Autodesk Fusion 360 part; units mm, degrees
sketch "Sketch1" plane through (0, 0, 0) normal (0, 1, 0) x (1, 0, 0)
  line L0 (0, 0) -> (39, 0)
  line L1 (0, 0) -> (-39, 0)
  line L2 (39, 0) -> (39, -36)
  line L3 (-39, -36) -> (39, -36)
  line L4 (-39, 0) -> (-49, -5.7735)
  line L5 (-39, 0) -> (1.8239, 0) construction
  line L6 (-49, -5.7735) -> (-49, -17.7735)
  line L7 (-49, -17.7735) -> (-39, -36)
  dimension "d1" = 39
  dimension "d2" = 39
  dimension "d4" = 36
  dimension "d5" = 36
  dimension "d8" = 12
extrude "Extrude1" add sketch "Sketch1" along normal mid plane 60
sketch "Sketch2" plane through (0, 0, 0) normal (0, 0, 1) x (1, 0, 0)
  line L0 (39, -30) -> (39, -12)
  line L1 (39, -12) -> (39, 12)
  line L2 (33, -30) -> (9, -30)
  line L3 (33, -12) -> (9, -12)
  line L4 (9, -12) -> (9, -30)
  line L5 (39, 12) -> (-3, 12)
  line L6 (39, -12) -> (-3, -12)
  line L7 (-3, -12) -> (-3, 12)
  dimension "d11" = 18
  dimension "d12" = 24
  dimension "d13" = 24
  dimension "d14" = 42
  dimension "d15" = 42
extrude "Extrude2" cut sketch "Sketch2" along normal blind 10 from surface at 30
sketch "Sketch3" plane through (0, 0, 0) normal (0, 0, 1) x (1, 0, 0)
  line L0 (27, -30) -> (3, -30)
  line L1 (27, -30) -> (27, -12)
  line L2 (3, -30) -> (3, -12)
  line L3 (3, -12) -> (27, -12)
  dimension "d20" = 24
  dimension "d21" = 18
  dimension "d22" = 18
extrude "Extrude3" cut sketch "Sketch3" along normal blind 30 from surface at 12
sketch "Sketch4" plane through (0, 0, 0) normal (0, 0, 1) x (1, 0, 0)
  line L0 (-3, 12) -> (-3, 24)
  line L1 (-3, 30) -> (-40, 30)
  line L2 (-40, 24) -> (-3, 24)
  line L3 (-40, 24) -> (-49.0656, 24)
  line L4 (-3, -24) -> (-49, -24)
  line L5 (-3, -24) -> (-3, -12)
  line L6 (-3, -12) -> (-3, 12)
  line L7 (-49.0656, 24) -> (-49, -24)
  dimension "d27" = 6
extrude "Extrude4" cut sketch "Sketch4" along normal blind 30 from surface at 12
sketch "Sketch5" plane through (0, 0, 0) normal (0, 1, 0) x (1, 0, 0)
  line L0 (-27, -12) -> (-3, -12)
  line L1 (-3, -12) -> (-3, -27)
  line L2 (-27, -12) -> (-3, -27)
  dimension "d34" = 24
  dimension "d35" = 15
extrude "Extrude5" cut sketch "Sketch5" against normal blind 35
sketch "Sketch6" plane through (0, 0, 0) normal (0, 1, 0) x (1, 0, 0)
  line L0 (-29, -30) -> (-11, -30)
  line L1 (-29, -30) -> (-29, -18)
  line L2 (-11, -30) -> (-11, -18)
  line L3 (-11, -18) -> (-29, -18)
  dimension "d41" = 18
  dimension "d42" = 12
  dimension "d43" = 12
extrude "Extrude6" cut sketch "Sketch6" along normal blind 35
Check sheet for the modelled part. Datum: model origin and axes. Units: mm. A direction names the side the tool comes from. Round coordinates to 2 decimals unless told otherwise and drop trailing zeros. Order: outer loops, then holes, each group sorted by start corner. A loop starts at its lowest first (then second) coordinate and runs counter-clockwise, first axis right, second up. Notation, with made-up numbers: (25, 36) -> (70, 36) arc R21 ccw to (70, 41) -> close; hole circle Ø6 at (49.5, -31). An arc over 180 degrees is marked (long way). Use CSV: the item, a comma, the result in double quotes.
(1) Cross-section at B-B (y = -18.5). Record the boundary of the cut face in (x, z).
Worked out:
outline,"(-49, 5.77) -> (-39, 0) -> (39, 0) -> (39, 36) -> (27, 36) -> (27, 12) -> (3, 12) -> (3, 36) -> (-3, 36) -> (-3, 12) -> (-49, 12) -> close"
(2) Cross-section at D-D (z = 23). Record the boundary of the cut face in (x, y).
Worked out:
outline,"(-46.13, -30) -> (-9.4, -30) -> (-9.4, -24) -> (-46.13, -24) -> close; (-46.13, 24) -> (-29, 24) -> (-29, 30) -> (-46.13, 30) -> close; (-11, 24) -> (-3, 24) -> (-3, -30) -> (3, -30) -> (3, -12) -> (27, -12) -> (27, -30) -> (39, -30) -> (39, 30) -> (-11, 30) -> close"
(3) Tool access check on faces 4 (the face through (-1, 0, 0)), 5 (the face through (18, 12, 33)), 6 (the face through (15, -21, 12)), 7 (the face through (-31, 24, 24)), 8 (the face through (-29, 27, 24)). Record the directions out of +Z, -Z, +X, -X, +Y, -Y that give a thin tool (end or side, any length) a straight path to the whole face; none if there is none.
Worked out:
face 4,"-Z, +X, -X, +Y, -Y"
face 5,"+Z, +X, -X"
face 6,"+Z, -Y"
face 7,"+Z, -X"
face 8,"+Y"
(4) Cross-section at A-A (z = 14). Record the boundary of the cut face in (x, y).
Worked out:
outline,"(-49, -30) -> (-23.8, -30) -> (-23.8, -24) -> (-49, -24) -> close; (-49, 24) -> (-3, 24) -> (-3, -30) -> (3, -30) -> (3, -12) -> (27, -12) -> (27, -30) -> (39, -30) -> (39, 30) -> (-49, 30) -> close"
(5) Depth check by flat-ended pin: pin 1 (6 mm diameter, centred on x = 23.5, z = 16.5, fed in from -Y); pin 2 (5.5 mm diameter, centred on y = -21, z = 19, fed in from -X); pin 3 (20 mm diameter, centred on x = 15.5, y = -21, fed in from +Z). Enter the tip coordinate at first touch or a pass-through.
Worked out:
pin 1,"y = -12"
pin 2,"x = -3"
pin 3,"z = 30"
(6) Cross-section at C-C (x = -15.5). Record the boundary of the cut face in (y, z).
Worked out:
outline,"(-30, 0) -> (30, 0) -> (30, 18) -> (24, 18) -> (24, 12) -> (-30, 12) -> close; (-30, 19.19) -> (-24, 19.19) -> (-24, 36) -> (-30, 36) -> close; (24, 30) -> (30, 30) -> (30, 36) -> (24, 36) -> close"
(7) Draft check along X on faces 1 (the face through (-44.07, -27.04, 26.76)), 2 (the face through (-20, 27, 30)), 3 (the face through (-6, 30, 18)). Enter one of: pulls with the +X half, pulls with the -X half, needs draft (parallel to the pull), parting line crosses it, or undercut.
Worked out:
face 1,"pulls with the -X half"
face 2,"undercut"
face 3,"needs draft"
(8) Material ranges on line 1 along X through (y, z) = (-23.5, 26); line 2 along Z through (x, y) = (-31, -2); line 3 along X through (y, z) = (1, 20.5), recorded low to high. Write a range as from..to.
Worked out:
line 1,"-3..3, 27..39"
line 2,"0..12"
line 3,"-3..39"
